Build history of the part. All positions in model axes, mm. A direction names the side the tool comes from. Round coordinates to 2 decimals unless told otherwise and drop trailing zeros. Order: outer loops, then holes, each group sorted by start corner. A loop starts at its lowest first (then second) coordinate and runs counter-clockwise, first axis right, second up. Notation, with made-up numbers: M -5,7.5 L 20,7.5 A24 cw 20,46.5 Z; hole C -23,-6 d5. An arc over 180 degrees is marked long. One line per item, written item: value. Start each with the question number.
Item 1: Band-saw the part on A-A, the plane y = 0. Write the cut outline in (x, z).
Item 2: Band-saw the part on D-D, the plane x = -11. Write the cut outline in (y, z).
Item 3: Pin check, flat tips, straight feed: pin 1 (4 mm diameter, centred on y = 13, z = 3, fed in from +X); pin 2 (6 mm diameter, centred on y = -5.5, z = -3, fed in from -X); pin 3 (6 mm diameter, centred on y = -3, z = 3, fed in from -X). Stop position of each tip, or through.
Item 4: Probe L1, parallel to Y at x = 0, z = -0.5; L2, parallel to Y at x = 0, z = -2.25; L3, parallel to Z at x = 14.5, y = 3. List the from-to ranges inside material, lowest first.
Item 5: Band-saw the part on C-C, the plane z = 0.25. Write the cut outline in (x, y), then the cut area to 3 significant figures.
Item 6: Tool access for faces 1 (the cylindrical face through (12.037, 4.991, 3.816)), 2 (the flat face through (3, -3, 6.35)), 3 (the flat face through (-13, -4, -1.352)): list every direction of +Z, -Z, +X, -X, +Y, -Y with a clear straight run to the whole face (end or side of a thin tool).
Item 7: Two-plate mould, pull along Y, no slides. Class faces 4 (the cylindrical face through (12.037, -4.991, -3.816)), 5 (the cylindrical face through (-3, 0, 0)), 6 (the flat face through (13, -4, 1.352)): +Y half, -Y half, draft (parallel to the pull), parting line (faces both ways), or undercut.
Autodesk Inventor part; units mm, degrees
ref_plane "YZ Plane" through (0, 0, 0) normal (1, 0, 0) x (0, 1, 0)
ref_plane "XZ Plane" through (0, 0, 0) normal (0, 1, 0) x (-1, 0, 0)
ref_plane "XY Plane" through (0, 0, 0) normal (0, 0, 1) x (1, 0, 0)
sketch "Sketch1" plane through (0, 0, 0) normal (0, 0, 1) x (1, 0, 0)
  circle A0 centre (0, 0) radius 13.0302
  circle A1 centre (0, 0) radius 3
  circle A2 centre (0, 0) radius 19.939
  dimension "d0" = 26.0604
  dimension "d1" = 6
  dimension "d2" = 39.878
extrude "Extrusion1" add sketch "Sketch1" along normal blind 6.35 contours A0
extrude "Extrusion2" add sketch "Sketch1" along normal blind 1.3525 contours A2
mirror "Mirror1" about plane through (0, 0, 0) normal (0, 0, -1)
properties part number "TensionerSprocket" material "Steel"
Output:
1. outline: M -19.94,-1.35 L -13.03,-1.35 L -13.03,-6.35 L -3,-6.35 L -3,6.35 L -13.03,6.35 L -13.03,1.35 L -19.94,1.35 Z; M 3,-6.35 L 13.03,-6.35 L 13.03,-1.35 L 19.94,-1.35 L 19.94,1.35 L 13.03,1.35 L 13.03,6.35 L 3,6.35 Z
2. outline: M -16.63,-1.35 L -6.98,-1.35 L -6.98,-6.35 L 6.98,-6.35 L 6.98,-1.35 L 16.63,-1.35 L 16.63,1.35 L 6.98,1.35 L 6.98,6.35 L -6.98,6.35 L -6.98,1.35 L -16.63,1.35 Z
3. pin 1: stops at x = 16.02
3. pin 2: stops at x = -19.71
3. pin 3: stops at x = -19.93
4. L1: y = -19.94 to -3, 3 to 19.94
4. L2: y = -13.03 to -3, 3 to 13.03
4. L3: z = -1.35 to 1.35
5. outline: C 0,0 d39.88; hole C 0,0 d6
5. area: 1,220 mm²
6. face 1: +Z
6. face 2: +Z, +X, -X, +Y, -Y
6. face 3: -Z
7. face 4: parting line
7. face 5: undercut
7. face 6: draft
